from build123d import *

# Parameters (mm, degrees)
F0_W         = 50.8
F0_H         = 18.3891410583
F1_DEPTH     = 3.175
F2_R         = 1.27
F3_DEPTH     = 25.4
F4_R         = 1.397
F5_DEPTH     = 2.54
F6_W         = 50.8
F6_H         = 29.8823560312
F7_DEPTH     = 4.826
F8_T1_DEPTH  = 33.401
F8_T6_DEPTH  = 55.2823560312
F8_T12_DEPTH = 55.2823560312
F8_T18_DEPTH = 55.2823560312
F8_T25_DEPTH = 55.2823560312
F8_T31_DEPTH = 55.2823560312
F8_T37_DEPTH = 55.2823560312
F8_T43_DEPTH = 55.2823560312
F8_T49_DEPTH = 55.2823560312
F8_T56_DEPTH = 55.2823560312
F8_T62_DEPTH = 55.2823560312
F9_T1_DEPTH  = 41.9355712549


# Not quite as in the source:
# - a fillet or chamfer that OpenCascade refuses, or shapes differently, is made with other operations: its cross-section is extruded or revolved along the edge and cut away or added


with BuildPart() as f1:
    # F0 (on Top) → F1 (new body)
    with BuildSketch(Plane.XY):
        Polygon((-25.4, -14.9411780156), (25.4, -14.9411780156), (25.4, -9.1945705292), (25.4, 9.1945705292), (25.4, 14.9411780156), (-25.4, 14.9411780156), (-25.4, 9.1945705292), (-25.4, -9.1945705292), align=None)
        with Locations((50.8, 0)):
            Rectangle(F0_W, F0_H)
        with Locations((-50.8, 0)):
            Rectangle(F0_W, F0_H)
    extrude(amount=F1_DEPTH)

    # F2 (on face) → F3 (cut)
    with BuildSketch(Plane.XY.offset(3.175)):
        with Locations((63.5, 0)):
            Circle(F2_R)
        with Locations((50.8, 0)):
            Circle(F2_R)
        with Locations((38.1, 0)):
            Circle(F2_R)
    extrude(amount=-F3_DEPTH, mode=Mode.SUBTRACT)

    # F4 (on face) → F5 (join)
    with BuildSketch(Plane.XY.offset(3.175)):
        with Locations((-68.6719441229, 0)):
            Circle(F4_R)
        with Locations((-55.9719441229, 0)):
            Circle(F4_R)
        with Locations((-43.2719441229, 0)):
            Circle(F4_R)
    extrude(amount=F5_DEPTH)

    # F6 (on face) → F7 (join)
    with BuildSketch(Plane.XY.offset(3.175)):
        Rectangle(F6_W, F6_H)
    extrude(amount=F7_DEPTH)

    # F8: fillet of radius 5.08 on 6 edges, made by hand

    # F8_s2 → F8_t1 (cut)
    with BuildSketch(Plane.XY.offset(-12.7)):
        with BuildLine():
            ThreePointArc((-20.32, 14.9411780156), (-23.9121024484, 13.453280464), (-25.4, 9.8611780156))
            Line((-25.4, 9.8611780156), (-25.4, 14.9411780156))
            Line((-25.4, 14.9411780156), (-20.32, 14.9411780156))
        make_face()
        with BuildLine():
            ThreePointArc((-20.32, -14.9411780156), (-23.9121024484, -13.453280464), (-25.4, -9.8611780156))
            Line((-25.4, -9.8611780156), (-25.4, -14.9411780156))
            Line((-25.4, -14.9411780156), (-20.32, -14.9411780156))
        make_face()
        with BuildLine():
            ThreePointArc((20.32, -14.9411780156), (23.9121024484, -13.453280464), (25.4, -9.8611780156))
            Line((25.4, -9.8611780156), (25.4, -14.9411780156))
            Line((25.4, -14.9411780156), (20.32, -14.9411780156))
        make_face()
        with BuildLine():
            ThreePointArc((20.32, 14.9411780156), (23.9121024484, 13.453280464), (25.4, 9.8611780156))
            Line((25.4, 9.8611780156), (25.4, 14.9411780156))
            Line((25.4, 14.9411780156), (20.32, 14.9411780156))
        make_face()
    extrude(amount=F8_T1_DEPTH, mode=Mode.SUBTRACT)


with BuildPart() as f8_tool4:
    # F8_s5 → F8_t6 (new body)
    with BuildSketch(Plane.XZ.offset(27.6411780156)):
        with BuildLine():
            ThreePointArc((25.4, 2.921), (23.9121024484, 6.5131024484), (20.32, 8.001))
            Line((20.32, 8.001), (25.4, 8.001))
            Line((25.4, 8.001), (25.4, 2.921))
        make_face()
    extrude(amount=-F8_T6_DEPTH)

    split(bisect_by=Plane.XY.offset(3.175), keep=Keep.BOTTOM)

    split(bisect_by=Plane.XZ.offset(9.1945705292), keep=Keep.TOP)


with BuildPart() as f1_1:
    add(f1.part)

    # F8_t3: cut F8_tool4
    add(f8_tool4.part, mode=Mode.SUBTRACT)


with BuildPart() as f8_tool10:
    # F8_s11 → F8_t12 (new body)
    with BuildSketch(Plane.XZ.offset(27.6411780156)):
        with BuildLine():
            ThreePointArc((25.4, 2.921), (23.9121024484, 6.5131024484), (20.32, 8.001))
            Line((20.32, 8.001), (25.4, 8.001))
            Line((25.4, 8.001), (25.4, 2.921))
        make_face()
    extrude(amount=-F8_T12_DEPTH)

    split(bisect_by=Plane.XY.offset(3.175), keep=Keep.TOP)

    split(bisect_by=Plane.XZ.offset(9.1945705292), keep=Keep.TOP)


with BuildPart() as f1_2:
    add(f1_1.part)

    # F8_t9: cut F8_tool10
    add(f8_tool10.part, mode=Mode.SUBTRACT)


with BuildPart() as f8_tool16:
    # F8_s17 → F8_t18 (new body)
    with BuildSketch(Plane.XZ.offset(27.6411780156)):
        with BuildLine():
            ThreePointArc((25.4, 2.921), (23.9121024484, 6.5131024484), (20.32, 8.001))
            Line((20.32, 8.001), (25.4, 8.001))
            Line((25.4, 8.001), (25.4, 2.921))
        make_face()
    extrude(amount=-F8_T18_DEPTH)

    split(bisect_by=Plane.XY.offset(3.175), keep=Keep.TOP)

    split(bisect_by=Plane.XZ.offset(-9.1945705292), keep=Keep.TOP)

    split(bisect_by=Plane.XZ.offset(9.1945705292), keep=Keep.BOTTOM)


with BuildPart() as f1_3:
    add(f1_2.part)

    # F8_t15: cut F8_tool16
    add(f8_tool16.part, mode=Mode.SUBTRACT)


with BuildPart() as f8_tool23:
    # F8_s24 → F8_t25 (new body)
    with BuildSketch(Plane.XZ.offset(27.6411780156)):
        with BuildLine():
            ThreePointArc((25.4, 2.921), (23.9121024484, 6.5131024484), (20.32, 8.001))
            Line((20.32, 8.001), (25.4, 8.001))
            Line((25.4, 8.001), (25.4, 2.921))
        make_face()
    extrude(amount=-F8_T25_DEPTH)

    split(bisect_by=Plane.XY.offset(3.175), keep=Keep.BOTTOM)

    split(bisect_by=Plane.XZ.offset(-9.1945705292), keep=Keep.BOTTOM)


with BuildPart() as f1_4:
    add(f1_3.part)

    # F8_t22: cut F8_tool23
    add(f8_tool23.part, mode=Mode.SUBTRACT)


with BuildPart() as f8_tool29:
    # F8_s30 → F8_t31 (new body)
    with BuildSketch(Plane.XZ.offset(27.6411780156)):
        with BuildLine():
            ThreePointArc((25.4, 2.921), (23.9121024484, 6.5131024484), (20.32, 8.001))
            Line((20.32, 8.001), (25.4, 8.001))
            Line((25.4, 8.001), (25.4, 2.921))
        make_face()
    extrude(amount=-F8_T31_DEPTH)

    split(bisect_by=Plane.XY.offset(3.175), keep=Keep.TOP)

    split(bisect_by=Plane.XZ.offset(-9.1945705292), keep=Keep.BOTTOM)


with BuildPart() as f1_5:
    add(f1_4.part)

    # F8_t28: cut F8_tool29
    add(f8_tool29.part, mode=Mode.SUBTRACT)


with BuildPart() as f8_tool35:
    # F8_s36 → F8_t37 (new body)
    with BuildSketch(Plane.XZ.offset(-27.6411780156)):
        with BuildLine():
            ThreePointArc((-20.32, 8.001), (-23.9121024484, 6.5131024484), (-25.4, 2.921))
            Line((-25.4, 2.921), (-25.4, 8.001))
            Line((-25.4, 8.001), (-20.32, 8.001))
        make_face()
    extrude(amount=F8_T37_DEPTH)

    split(bisect_by=Plane.XZ.offset(-9.1945705292), keep=Keep.BOTTOM)

    split(bisect_by=Plane.XY.offset(3.175), keep=Keep.TOP)


with BuildPart() as f1_6:
    add(f1_5.part)

    # F8_t34: cut F8_tool35
    add(f8_tool35.part, mode=Mode.SUBTRACT)


with BuildPart() as f8_tool41:
    # F8_s42 → F8_t43 (new body)
    with BuildSketch(Plane.XZ.offset(-27.6411780156)):
        with BuildLine():
            ThreePointArc((-20.32, 8.001), (-23.9121024484, 6.5131024484), (-25.4, 2.921))
            Line((-25.4, 2.921), (-25.4, 8.001))
            Line((-25.4, 8.001), (-20.32, 8.001))
        make_face()
    extrude(amount=F8_T43_DEPTH)

    split(bisect_by=Plane.XZ.offset(-9.1945705292), keep=Keep.BOTTOM)

    split(bisect_by=Plane.XY.offset(3.175), keep=Keep.BOTTOM)


with BuildPart() as f1_7:
    add(f1_6.part)

    # F8_t40: cut F8_tool41
    add(f8_tool41.part, mode=Mode.SUBTRACT)


with BuildPart() as f8_tool47:
    # F8_s48 → F8_t49 (new body)
    with BuildSketch(Plane.XZ.offset(-27.6411780156)):
        with BuildLine():
            ThreePointArc((-20.32, 8.001), (-23.9121024484, 6.5131024484), (-25.4, 2.921))
            Line((-25.4, 2.921), (-25.4, 8.001))
            Line((-25.4, 8.001), (-20.32, 8.001))
        make_face()
    extrude(amount=F8_T49_DEPTH)

    split(bisect_by=Plane.XZ.offset(-9.1945705292), keep=Keep.TOP)

    split(bisect_by=Plane.XY.offset(3.175), keep=Keep.TOP)

    split(bisect_by=Plane.XZ.offset(9.1945705292), keep=Keep.BOTTOM)


with BuildPart() as f1_8:
    add(f1_7.part)

    # F8_t46: cut F8_tool47
    add(f8_tool47.part, mode=Mode.SUBTRACT)


with BuildPart() as f8_tool54:
    # F8_s55 → F8_t56 (new body)
    with BuildSketch(Plane.XZ.offset(-27.6411780156)):
        with BuildLine():
            ThreePointArc((-20.32, 8.001), (-23.9121024484, 6.5131024484), (-25.4, 2.921))
            Line((-25.4, 2.921), (-25.4, 8.001))
            Line((-25.4, 8.001), (-20.32, 8.001))
        make_face()
    extrude(amount=F8_T56_DEPTH)

    split(bisect_by=Plane.XY.offset(3.175), keep=Keep.TOP)

    split(bisect_by=Plane.XZ.offset(9.1945705292), keep=Keep.TOP)


with BuildPart() as f1_9:
    add(f1_8.part)

    # F8_t53: cut F8_tool54
    add(f8_tool54.part, mode=Mode.SUBTRACT)


with BuildPart() as f8_tool60:
    # F8_s61 → F8_t62 (new body)
    with BuildSketch(Plane.XZ.offset(-27.6411780156)):
        with BuildLine():
            ThreePointArc((-20.32, 8.001), (-23.9121024484, 6.5131024484), (-25.4, 2.921))
            Line((-25.4, 2.921), (-25.4, 8.001))
            Line((-25.4, 8.001), (-20.32, 8.001))
        make_face()
    extrude(amount=F8_T62_DEPTH)

    split(bisect_by=Plane.XY.offset(3.175), keep=Keep.BOTTOM)

    split(bisect_by=Plane.XZ.offset(9.1945705292), keep=Keep.TOP)


with BuildPart() as f1_10:
    add(f1_9.part)

    # F8_t59: cut F8_tool60
    add(f8_tool60.part, mode=Mode.SUBTRACT)

    # F9: fillet of radius 5.08 on 2 edges, made by hand

    # F9_s2 → F9_t1 (cut)
    with BuildSketch(Plane.XZ.offset(-20.9677856274)):
        with BuildLine():
            ThreePointArc((71.4907139607, 3.175), (74.3305202921, 2.3071134838), (76.2, 0))
            Line((76.2, 0), (76.2, 3.175))
            Line((76.2, 3.175), (71.4907139607, 3.175))
        make_face()
        with BuildLine():
            ThreePointArc((-76.2, 0), (-74.3305202921, 2.3071134838), (-71.4907139607, 3.175))
            Line((-71.4907139607, 3.175), (-76.2, 3.175))
            Line((-76.2, 3.175), (-76.2, 0))
        make_face()
    extrude(amount=F9_T1_DEPTH, mode=Mode.SUBTRACT)


solid = f1_10.part
For this review, take the finished solid that the model builds, in its own axes (mm). A direction names the side the tool comes from. Give positions to 0.01 mm unless a question says otherwise; leave off trailing zeros. Loops run counter-clockwise (first coordinate to the right, second up) from the corner with the lowest first, then second, coordinate; pieces in that order, holes last.
Item 1: Draft analysis for pull direction X (two halves, no side actions). For faces 1 (the flat face through (48, 0, 3.175)), 2 (the cylindrical face through (36.83, 0.06, 1.61)), 3 (the cylindrical face through (74.295, 0.129, 2.331)), state which applies: +X half, -X half, draft (parallel to the pull), parting line (faces both ways), or undercut.
Item 2: Take a section at B-B, the plane x = -60.5. State the section outline as (y, z) points (3 decimals).
Item 3: Tool access review of faces 4 (the flat face through (50, -9.195, 2)), 5 (the flat face through (-43, 0, 5.715)), 6 (the flat face through (-51, 9.195, 2)): name each direction out of +Z, -Z, +X, -X, +Y, -Y from which nothing blocks a thin tool from reaching the whole face with its end or side.
Item 4: For line 1 along Y through (x, z) = (38.1, 2); line 2 along Z through (x, y) = (44, 0) (3 decimals); line 3 along Z through (x, y) = (-20.5, 12.25), list the stretches that pass through material, from the lowest coordinate up.
Item 5: Insertion check: pin 1 (1.5 mm diameter, centred on x = -44, z = 7, fed in from -Y); pin 2 (1.4 mm diameter, centred on x = -44, y = 0, fed in from +Z) (3 decimals); pin 3 (2.5 mm diameter, centred on x = 44, z = 1.5, fed in from -Y); pin 4 (12 mm diameter, centred on x = 44.5, y = 7, fed in from +Z) (3 decimals). Each pin has a flat end and moves straight along its axis. Give the tip position at first contact, or say it passes through.
Item 6: Take a section at A-A, the plane x = 63.5. State the section outline as (y, z) points (3 decimals), and give its area (3 significant figures).
Item 7: Take a section at C-C, the plane y = 13. State the section outline as (x, z) points, and give its area (3 significant figures).
Calculated:
1. face 1: draft
1. face 2: undercut
1. face 3: +X half
2. outline: (-9.195, 0) - (9.195, 0) - (9.195, 3.175) - (-9.195, 3.175) - close
3. face 4: +Z, -Z, +X, -Y
3. face 5: +Z, -X, +Y, -Y
3. face 6: +Z, -Z, -X, +Y
4. line 1: y = -9.19 to -1.27, 1.27 to 9.19
4. line 2: z = 0 to 3.175
4. line 3: z = 0 to 8
5. pin 1: passes through
5. pin 2: stops at z = 5.715
5. pin 3: stops at y = -9.19
5. pin 4: stops at z = 3.175
6. outline: (-9.195, 0) - (-1.27, 0) - (-1.27, 3.175) - (-9.195, 3.175) - close; (1.27, 0) - (9.195, 0) - (9.195, 3.175) - (1.27, 3.175) - close
6. area: 50.3 mm2
7. outline: (-24.31, 0) - (24.31, 0) - (24.31, 6.06) arc R5.08 ccw to (20.32, 8) - (-20.32, 8) arc R5.08 ccw to (-24.31, 6.06) - close
7. area: 384 mm2
